The listing builds one solid part. Answer for the finished solid, in the listing's coordinates (mm). Face numbers are marked on the shaded views. Coordinates: 2 decimals unless noted, no trailing zeros. Write each loop counter-clockwise with the first axis right and the second up, starting at its lowest first coordinate (ties: lowest second). Pieces come first, ordered by that corner, then holes. Notation, with made-up numbers: M -12.75,1.25 L 35.25,1.25 A12 ccw 35.25,18.25 Z; hole C 59.5,32.5 d5. An arc over 180 degrees is marked long. Answer as CSV lines item,"result".
```python
from build123d import *

# Parameters (mm, degrees)
EXTRUDE_1_DEPTH          = 10
EXTRUDE_1_DEPTH_BACK     = 10
SKETCH_1_R               = 8
SKETCH_1_R_2             = 6
SKETCH_2_R               = 14
SKETCH_2_R_2             = 12.5
EXTRUDE_2_DEPTH          = 12.5
CUT_EXTRUDE_1_DEPTH      = 35.543451059
CUT_EXTRUDE_1_DEPTH_BACK = 35.543451059
SKETCH_3_R               = 12.5
CUT_EXTRUDE_START        = -14.034144001
CUT_EXTRUDE_2_OUTLINE_R  = 6
CUT_EXTRUDE_2_DEPTH      = 3.034143808


# Read off the part's stored shape, not the designer's step: the extrude step
with BuildPart() as part:
    # Sketch 1 → Extrude 1 (new, two sides: drawn at the far end of the back side and taken through both)
    with BuildSketch(Plane(origin=(0, 0, 0), x_dir=(1, 0, 0), z_dir=(0, 1, 0)).offset(-EXTRUDE_1_DEPTH_BACK)):
        with Locations(Location((0, 0, 0), (0, 0, 270))):
            Circle(SKETCH_1_R)
        with Locations(Location((0, 0, 0), (0, 0, 270))):
            Circle(SKETCH_1_R_2, mode=Mode.SUBTRACT)
    extrude(amount=EXTRUDE_1_DEPTH + EXTRUDE_1_DEPTH_BACK)

    # Sketch 2 → Extrude 2 (add, symmetric)
    with BuildSketch(Plane(origin=(0, 0, 0), x_dir=(0, 0, -1), z_dir=(1, 0, 0))):
        with Locations((0, 15)):
            Circle(SKETCH_2_R)
        with Locations((0, 15)):
            Circle(SKETCH_2_R_2, mode=Mode.SUBTRACT)
    extrude(amount=EXTRUDE_2_DEPTH, both=True)

    # Sketch 3 → Cut-Extrude 1 (cut, two sides: drawn at the far end of the back side and taken through both)
    with BuildSketch(Plane(origin=(0, 0, 0), x_dir=(0, 0, -1), z_dir=(1, 0, 0)).offset(-CUT_EXTRUDE_1_DEPTH_BACK)):
        with Locations((0, 15)):
            Circle(SKETCH_3_R)
    extrude(amount=CUT_EXTRUDE_1_DEPTH + CUT_EXTRUDE_1_DEPTH_BACK, mode=Mode.SUBTRACT)

    # Cut-Extrude 2 outline → Cut-Extrude 2 (cut)
    with BuildSketch(Plane.XZ.offset(10).offset(CUT_EXTRUDE_START)):
        Circle(CUT_EXTRUDE_2_OUTLINE_R)
    extrude(amount=CUT_EXTRUDE_2_DEPTH, mode=Mode.SUBTRACT)


solid = part.part
```
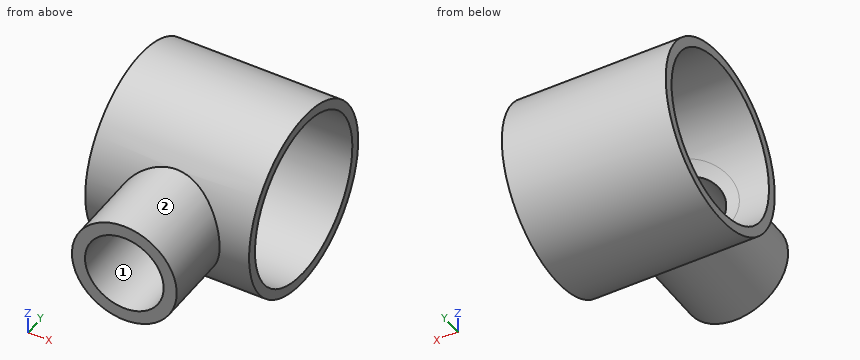
Q1. Find section D-D (x = -11). Give the vertices of the cut face in (y, z).
Output:
outline,"C 15,0 d28; hole C 15,0 d25"
Q2. Find section B-B (y = 15). Give the vertices of the cut face in (x, z).
Output:
outline,"M -12.5,-14 L 12.5,-14 L 12.5,-12.5 L -12.5,-12.5 Z; M -12.5,12.5 L 12.5,12.5 L 12.5,14 L -12.5,14 Z"
Q3. Find section A-A (z = 0). Give the vertices of the cut face in (x, y), and give its area (3 significant figures).
Output:
outline,"M -12.5,1 L -8,1 L -8,-10 L -6,-10 L -6,2.5 L -12.5,2.5 Z; M -12.5,27.5 L 12.5,27.5 L 12.5,29 L -12.5,29 Z; M 6,-10 L 8,-10 L 8,1 L 12.5,1 L 12.5,2.5 L 6,2.5 Z"
area,"101 mm2"
Q4. Straight lines are drawn through the part: line 1 (Y direction, x = -9.25, z = 0.5); line 2 (Z direction, x = 0, y = -2.75); line 3 (Y direction, x = 4, z = 0). For each, find the intervals that lie inside material, in ascending order.
Output:
line 1,"1.01 to 2.51, 27.49 to 28.99"
line 2,"-8 to -6, 6 to 8"
line 3,"27.5 to 29"
Q5. Flat-ended cylindrical pins translate along their axes: pin 1 Ø1 at (y, z) = (24.5, 4.5) entering from -X; pin 2 Ø2 at (y, z) = (-5.5, 4.5) entering from +X; pin 3 Ø1 at (x, y) = (-6.5, 1) entering from -Z; pin 4 Ø5 at (x, z) = (-6, 10.5) entering from -Y. Find the tip coordinate at first contact, or state that the pin passes through.
Output:
pin 1,"through"
pin 2,"x = 7.19"
pin 3,"z = -5.29"
pin 4,"y = 3.51"
Q6. Find section C-C (z = 12). Give the vertices of the cut face in (x, y), and give its area (3 significant figures).
Output:
outline,"M -12.5,7.79 L 12.5,7.79 L 12.5,11.5 L -12.5,11.5 Z; M -12.5,18.5 L 12.5,18.5 L 12.5,22.21 L -12.5,22.21 Z"
area,"186 mm2"
Q7. The mould has two halves that part along X. Classify the marked faces 1 and 2: pulls with the +X half, pulls with the -X half, needs draft (parallel to the pull), parting line crosses it, or undercut.
Output:
face 1,"undercut"
face 2,"parting line crosses it"
